Verification items for this drawing (mm, ordinates from the low corner). A direction names the side the tool comes from. Round coordinates to 2 decimals unless told otherwise and drop trailing zeros. Loops run counter-clockwise (first coordinate to the right, second up) from the corner with the lowest first, then second, coordinate; pieces in that order, holes last. Notation, with made-up numbers: (14, 68) -> (36, 68) arc R27 cw to (36, 86) -> close; hole circle Ø7 at (12, 58.5). An arc over 180 degrees is marked (long way). One line per question, with ' | ' between items.
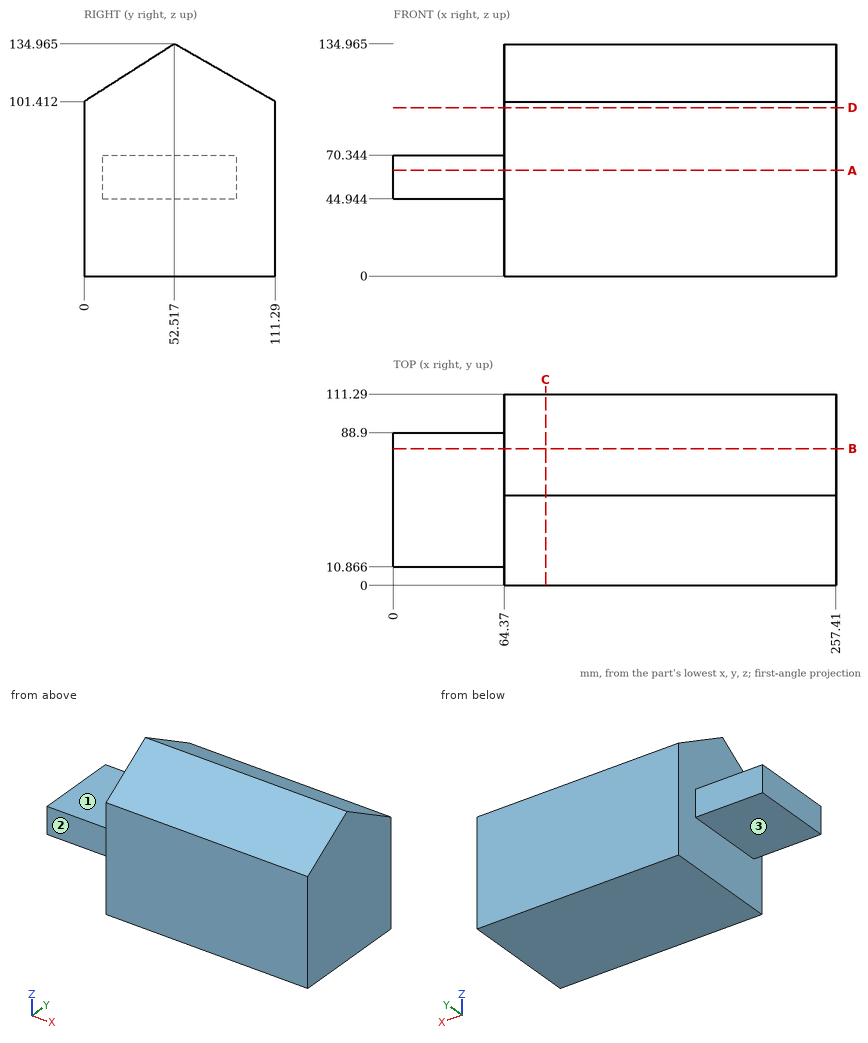
(1) Sectioned sample at A-A, the plane z = 61.5. Record the cut outline in (x, y) (1 decimal), and give its area (3 significant figures).
Answer:
outline: (0, 10.9) -> (64.4, 10.9) -> (64.4, 0) -> (257.4, 0) -> (257.4, 111.3) -> (64.4, 111.3) -> (64.4, 88.9) -> (0, 88.9) -> close | area: 26,500 mm2
(2) Scan lines: probe 1 along Z at (x, y) = (28, 38); probe 2 along X at (y, z) = (58, 11); probe 3 along Z at (x, y) = (86, 98.5) (1 decimal). Record each from-to range of solid material in increasing order.
Answer:
probe 1: z = 44.94 to 70.34 | probe 2: x = 64.37 to 257.41 | probe 3: z = 0 to 108.7
(3) Sectioned sample at D-D, the plane z = 98. Record the cut outline in (x, y).
Answer:
outline: (64.37, 0) -> (257.41, 0) -> (257.41, 111.29) -> (64.37, 111.29) -> close
(4) Sectioned sample at B-B, the plane y = 79.5. Record the cut outline in (x, z).
Answer:
outline: (0, 44.94) -> (64.37, 44.94) -> (64.37, 0) -> (257.41, 0) -> (257.41, 119.56) -> (64.37, 119.56) -> (64.37, 70.34) -> (0, 70.34) -> close
(5) Sectioned sample at C-C, the plane x = 88.5. Record the cut outline in (y, z) (1 decimal), and give its area (3 significant figures).
Answer:
outline: (0, 0) -> (111.3, 0) -> (111.3, 101.4) -> (52.5, 135) -> (0, 101.4) -> close | area: 13,200 mm2
(6) Go/stop test with flat-tipped pins: pin 1 (10 mm diameter, centred on x = 75.5, z = 91.5, fed in from -Y); pin 2 (6 mm diameter, centred on x = 164, y = 39, fed in from +Z) (1 decimal); pin 3 (12 mm diameter, centred on y = 44.5, z = 82, fed in from -X); pin 4 (2 mm diameter, centred on x = 175, y = 73, fed in from +Z). Record where each tip stops, or that it passes through.
Answer:
pin 1: stops at y = 0 | pin 2: stops at z = 128.2 | pin 3: stops at x = 64.37 | pin 4: stops at z = 123.84
(7) Set-up check for the marked faces 1, 2 and 3: record each of +Z, -Z, +X, -X, +Y, -Y from which the full face is reachable in a straight line by a thin tool's end or side.
Answer:
face 1: +Z, -X, +Y, -Y | face 2: +Z, -Z, -X, -Y | face 3: -Z, -X, +Y, -Y
